Job drawing, mm, ordinate dimensions from the low corner. One solid piece. A direction names the side the tool comes from. Give positions to 0.01 mm unless a question says otherwise; leave off trailing zeros. Write each loop counter-clockwise with the first axis right and the second up, starting at its lowest first coordinate (ties: lowest second). Pieces come first, ordered by that corner, then holes. Notation, with made-up numbers: (36.5, -1) - (56.5, -1) arc R38 ccw to (56.5, 38) - close; hole circle Ø2 at (76.5, 44.25). An arc over 180 degrees is marked (long way). Answer as a JSON object with one key per item and string values.
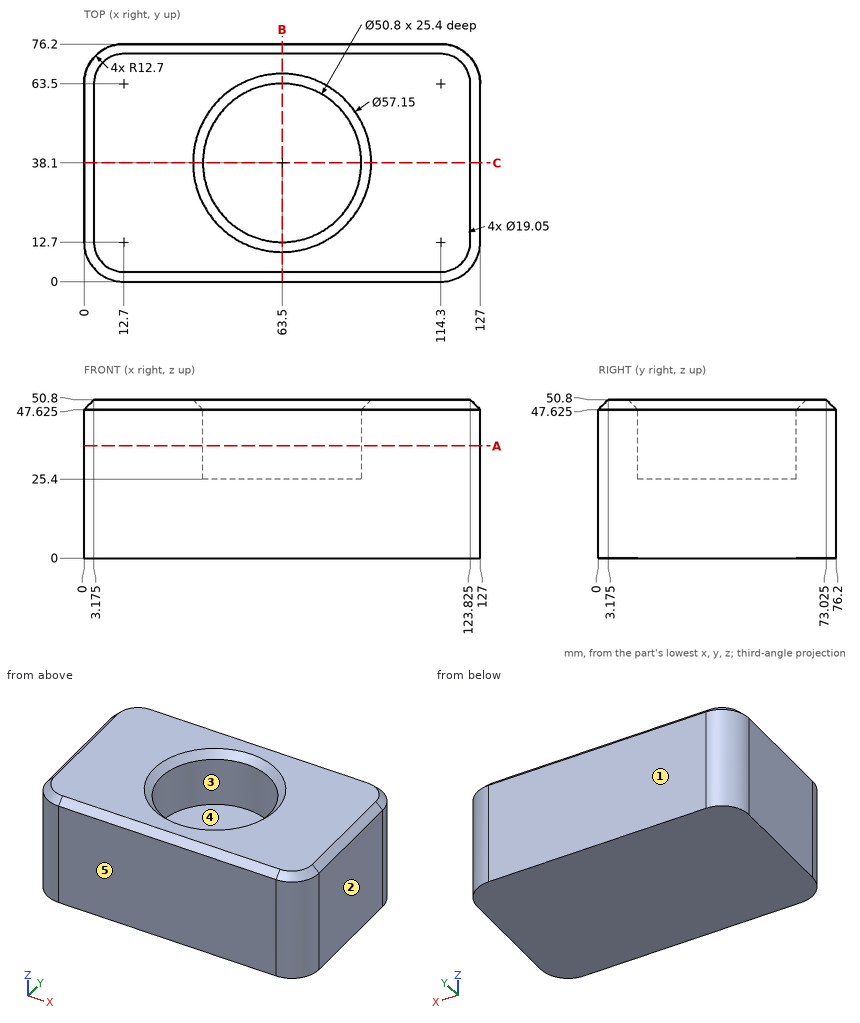
Item 1: Cut at C-C (y = 38.1). Give the cut face in (x, z) (3 decimals), and give its area (3 significant figures).
Entries:
{"outline": "(0, 0) - (127, 0) - (127, 47.625) - (123.825, 50.8) - (92.075, 50.8) - (88.9, 47.625) - (88.9, 25.4) - (38.1, 25.4) - (38.1, 47.625) - (34.925, 50.8) - (3.175, 50.8) - (0, 47.625) - close", "area": "5,140 mm2"}
Item 2: Mould opens along Y. For the marked faces 1, 2 and 3 say: +Y half, -Y half, draft (parallel to the pull), parting line (faces both ways), or undercut.
Entries:
{"face 1": "+Y half", "face 2": "draft", "face 3": "undercut"}
Item 3: Cut at B-B (x = 63.5). Give the cut face in (y, z) (3 decimals), and give its area (3 significant figures).
Entries:
{"outline": "(0, 0) - (76.2, 0) - (76.2, 47.625) - (73.025, 50.8) - (66.675, 50.8) - (63.5, 47.625) - (63.5, 25.4) - (12.7, 25.4) - (12.7, 47.625) - (9.525, 50.8) - (3.175, 50.8) - (0, 47.625) - close", "area": "2,560 mm2"}
Item 4: Which spindle directions (+Z, -Z, +X, -X, +Y, -Y) get a long thin tool onto all of the face, cutting with end or side? Do the marked faces 4 and 5. Say none if no direction does.
Entries:
{"face 4": "+Z", "face 5": "+Z, -Z, +X, -X, -Y"}
Item 5: Cut at A-A (z = 36). Give the cut face in (x, y).
Entries:
{"outline": "(0, 12.7) arc R12.7 ccw to (12.7, 0) - (114.3, 0) arc R12.7 ccw to (127, 12.7) - (127, 63.5) arc R12.7 ccw to (114.3, 76.2) - (12.7, 76.2) arc R12.7 ccw to (0, 63.5) - close; hole circle Ø50.8 at (63.5, 38.1)"}
Item 6: Probe line 1 (Y direction, x = 63.5, z = 37.75); line 2 (X direction, y = 38, z = 33); line 3 (X direction, y = 50, z = 27.5). List the from-to ranges inside material, lowest first. Write a range as from..to.
Entries:
{"line 1": "0..12.7, 63.5..76.2", "line 2": "0..38.1, 88.9..127", "line 3": "0..41.06, 85.94..127"}
